Input: part model. Units: mm. Frame: model coordinates. A direction names the side the tool comes from. Coordinates: 2 decimals unless noted, no trailing zeros. Order: outer loops, then holes, each group sorted by start corner. A loop starts at its lowest first (then second) coordinate and runs counter-clockwise, first axis right, second up. Notation, with made-up numbers: M 5,77 L 56,77 A6 ccw 56,84 Z; hole C -3,87.5 d11. An arc over 180 degrees is marked long. Answer in a Markdown table with one row per item.
from build123d import *

# Parameters (mm, degrees)
SKETCH1_W                                            = 60
SKETCH1_H                                            = 55
BOSS_EXTRUDE1_DEPTH                                  = 17.5
SKETCH2_W                                            = 20
SKETCH2_H                                            = 45
SKETCH2_H_2                                          = 40
CUT_EXTRUDE1_DEPTH                                   = 54.677276384
M4_TAPPED_HOLE1_D                                    = 3.3
CBORE_FOR_M4_HEXAGON_SOCKET_HEAD_CAP_SCR_D           = 4.5
CBORE_FOR_M4_HEXAGON_SOCKET_HEAD_CAP_SCR_CBORE_D     = 8
CBORE_FOR_M4_HEXAGON_SOCKET_HEAD_CAP_SCR_CBORE_DEPTH = 4.6
CHAMFER1_SIZE                                        = 5
CHAMFER2_START                                       = 25.980762114
CHAMFER2_OUTLINE_W                                   = 15
CHAMFER2_OUTLINE_H                                   = 17
CHAMFER2_DEPTH                                       = 7.019237886
CHAMFER3_START                                       = -33
CHAMFER3_OUTLINE_W                                   = 15
CHAMFER3_OUTLINE_H                                   = 17
CHAMFER3_DEPTH                                       = 7.019237886


with BuildPart() as part:
    # Sketch1 → Boss-Extrude1 (new, symmetric)
    with BuildSketch(Plane(origin=(0, 0, 0), x_dir=(1, 0, 0), z_dir=(0, 1, 0))):
        Rectangle(SKETCH1_W, SKETCH1_H)
    extrude(amount=BOSS_EXTRUDE1_DEPTH, both=True)

    # Sketch2 → Cut-Extrude1 (cut, through all)
    with BuildSketch(Plane(origin=(0, 17.5, 0), x_dir=(1, 0, 0), z_dir=(0, 1, 0))):
        with Locations((20, 5)):
            Rectangle(SKETCH2_W, SKETCH2_H)
        with Locations((-20, -7.5)):
            Rectangle(SKETCH2_W, SKETCH2_H_2)
    extrude(amount=-CUT_EXTRUDE1_DEPTH, mode=Mode.SUBTRACT)

    # M4 Tapped Hole1 (through all)
    with Locations(Plane(origin=(0, 0, 17.5), x_dir=(-1, 0, 0), z_dir=(0, 0, -1))):
        with Locations((-20, 10), (-20, -10)):
            Hole(M4_TAPPED_HOLE1_D / 2)

    # CBORE for M4 Hexagon socket head cap screws1 (through all)
    with Locations(Plane(origin=(0, 0, -27.5), x_dir=(-1, 0, 0), z_dir=(0, 0, -1))):
        with Locations((20, 10), (20, -10)):
            CounterBoreHole(CBORE_FOR_M4_HEXAGON_SOCKET_HEAD_CAP_SCR_D / 2, CBORE_FOR_M4_HEXAGON_SOCKET_HEAD_CAP_SCR_CBORE_D / 2, CBORE_FOR_M4_HEXAGON_SOCKET_HEAD_CAP_SCR_CBORE_DEPTH)

    # Chamfer1
    chamfer1_edges = [part.edges().sort_by_distance(p)[0] for p in [
        (30, 17.5, 22.5),
        (-30, 17.5, -20),
        (30, -17.5, 22.5),
        (-30, -17.5, -20),
    ]]
    chamfer(chamfer1_edges, length=CHAMFER1_SIZE)

    # Chamfer2: read off the stored shape, not the designer's step
    # Chamfer2 outline → Chamfer2 (cut)
    with BuildSketch(Plane(origin=(0, 0, 0), x_dir=(0.8164965809277258, 0.40824829046386313, 0.40824829046386313), z_dir=(0.5773502691896258, -0.5773502691896258, -0.5773502691896258)).offset(CHAMFER2_START)):
        with Locations((-12.5, -7.5)):
            Rectangle(CHAMFER2_OUTLINE_W, CHAMFER2_OUTLINE_H)
    chamfer2 = extrude(amount=CHAMFER2_DEPTH, mode=Mode.SUBTRACT)

    # Chamfer3: read off the stored shape, not the designer's step
    # Chamfer3 outline → Chamfer3 (cut)
    with BuildSketch(Plane(origin=(0, 0, 0), x_dir=(0.8164965809277258, -0.40824829046386313, 0.40824829046386313), z_dir=(0.5773502691896258, 0.5773502691896258, -0.5773502691896258)).offset(CHAMFER3_START)):
        with Locations((12.5, -7.5)):
            Rectangle(CHAMFER3_OUTLINE_W, CHAMFER3_OUTLINE_H)
    chamfer3 = extrude(amount=CHAMFER3_DEPTH, mode=Mode.SUBTRACT)

    # Mirror1: Chamfer2, Chamfer3 across plane
    add(chamfer2.mirror(Plane.ZX), mode=Mode.SUBTRACT)
    add(chamfer3.mirror(Plane.ZX), mode=Mode.SUBTRACT)


solid = part.part
1) Reachability of faces 1 (the face through (-10, 0, 8)), 2 (the face through (6, -15, -24)), 3 (the face through (-16.8, -12.4, -25.2)), 4 (the face through (-6.2, -14.5, 24.3)), 5 (the face through (20, 0, 17.5)) from +Z, -Z, +X, -X, +Y, -Y: full face, straight path, thin tool, end or side. Return the list, or none.
Resolved:
| item | result |
|---|---|
| face 1 | +Z, -X, +Y, -Y |
| face 2 | -Z, +X, -Y |
| face 3 | -Z |
| face 4 | +Z, -X, -Y |
| face 5 | -Z, +X, +Y, -Y |
2) Material intervals for probe 1 along Y at (x, z) = (20, 24.25); probe 2 along Y at (x, z) = (-20, -19); probe 3 along Z at (x, y) = (26, 10.5), sorted ascending.
Resolved:
| item | result |
|---|---|
| probe 1 | y = -17.5 to -11.65, -8.35 to 8.35, 11.65 to 17.5 |
| probe 2 | y = -17.5 to -12.25, -7.75 to 7.75, 12.25 to 17.5 |
| probe 3 | z = 17.5 to 27.5 |
3) Cut plane C-C, the plane z = -15.5. Output: boundary loops of the cut face in (x, y), and give its area (3 significant figures).
Resolved:
| item | result |
|---|---|
| outline | M -30,-12.5 L -25,-17.5 L 10,-17.5 L 10,17.5 L -25,17.5 L -30,12.5 Z; hole C -20,-10 d4.5; hole C -20,10 d4.5 |
| area | 1,340 mm2 |
4) Cut plane A-A, the plane x = -20. Output: boundary loops of the cut face in (y, z).
Resolved:
| item | result |
|---|---|
| outline | M -17.5,-27.5 L -14,-27.5 L -14,-22.9 L -12.25,-22.9 L -12.25,-12.5 L -17.5,-12.5 Z; M -7.75,-22.9 L -6,-22.9 L -6,-27.5 L 6,-27.5 L 6,-22.9 L 7.75,-22.9 L 7.75,-12.5 L -7.75,-12.5 Z; M 12.25,-22.9 L 14,-22.9 L 14,-27.5 L 17.5,-27.5 L 17.5,-12.5 L 12.25,-12.5 Z |
5) Cut plane B-B, the plane y = 10. Output: boundary loops of the cut face in (x, z).
Resolved:
| item | result |
|---|---|
| outline | M -30,-27.5 L -24,-27.5 L -24,-22.9 L -22.25,-22.9 L -22.25,-12.5 L -30,-12.5 Z; M -17.75,-22.9 L -16,-22.9 L -16,-27.5 L 7.5,-27.5 L 10,-25 L 10,17.5 L 18.35,17.5 L 18.35,27.5 L -7.5,27.5 L -10,25 L -10,-12.5 L -17.75,-12.5 Z; M 21.65,17.5 L 30,17.5 L 30,27.5 L 21.65,27.5 Z |
6) Contact query for flat-ended pins moving along their axis: pin 1 (5 mm diameter, centred on y = 4, z = -3, fed in from -X); pin 2 (7 mm diameter, centred on x = -20, y = 10, fed in from -Z); pin 3 (10.5 mm diameter, centred on y = 5, z = -6, fed in from +X). Output: stop coordinate, or through.
Resolved:
| item | result |
|---|---|
| pin 1 | stops at x = -10 |
| pin 2 | stops at z = -22.9 |
| pin 3 | stops at x = 10 |
7) Cut plane D-D, the plane y = -3. Output: boundary loops of the cut face in (x, z), and give its area (3 significant figures).
Resolved:
| item | result |
|---|---|
| outline | M -30,-27.5 L 10,-27.5 L 10,17.5 L 30,17.5 L 30,27.5 L -10,27.5 L -10,-12.5 L -30,-12.5 Z |
| area | 1,600 mm2 |
8) Mould query, pull axis X, two halves, no side actions, for faces 6 (the face through (0, -17.5, 0)), 7 (the face through (-6.2, 14.5, 24.3)), 8 (the face through (-18.79, 11.897, -17.627)). Classes: +X half, -X half, draft (parallel to the pull), parting line (faces both ways), or undercut.
Resolved:
| item | result |
|---|---|
| face 6 | draft |
| face 7 | -X half |
| face 8 | undercut |
